The listing builds one solid part. Answer for the finished solid, in the listing's coordinates (mm). A direction names the side the tool comes from. Round coordinates to 2 decimals unless told otherwise and drop trailing zeros. Write each loop counter-clockwise with the first axis right and the second up, starting at its lowest first coordinate (ties: lowest second). Pieces come first, ordered by that corner, then holes.
(1) A cutting plane is placed at C-C, the plane z = -40. Give the vertices of the cut face in (x, y), and give its area (3 significant figures).
(2) A cutting plane is placed at A-A, the plane y = 8. Give the vertices of the cut face in (x, z).
(3) Find the intervals of material crossed by probe 1 along Y at (x, z) = (42.5, 11); probe 2 along Y at (x, z) = (-42.5, -34.5); probe 3 along X at (y, z) = (24.5, 4), in increasing order.
(4) A cutting plane is placed at B-B, the plane z = -11. Give the vertices of the cut face in (x, y).
(5) A cutting plane is placed at D-D, the plane x = 0. Give the vertices of the cut face in (y, z).
(6) Each of these flat-tipped pins is pushed along its axis until it touches: pin 1 Ø6 at (y, z) = (5.5, 10) entering from +X; pin 2 Ø4 at (x, y) = (-41.5, 8) entering from +Z; pin 3 Ø4 at (x, y) = (-38, 13) entering from +Z; pin 4 Ø10.5 at (x, y) = (-44, 24.5) entering from +Z. Where does it stop, or does it pass through?
(7) For faces 4 (the face through (-44, 29.5, -11)), 5 (the face through (9.76, 14.79, 20)), 6 (the face through (36.3, 9.95, 8.31)), determine the directions among +Z, -Z, +X, -X, +Y, -Y from which every point of the face is accessible in a straight line to the end or side of a thin tool.
(8) The mould has two halves that part along Y. Classify faces 1 (the face through (43, 15, 14)), 2 (the face through (36.3, 23.95, 8.31)), 3 (the face through (-42.55, 0.49, 13.73)): +Y half, -Y half, draft (parallel to the pull), parting line (faces both ways), or undercut.
from build123d import *

# Parameters (mm, degrees)
SKETCH1_R               = 32.5
SKETCH1_R_2             = 6
BOSS_EXTRUDE1_DEPTH     = 30
CUT_EXTRUDE1_START      = -0.5
CUT_EXTRUDE1_DEPTH      = 0.5
SKETCH3_R               = 4.5
CUT_EXTRUDE2_DEPTH      = 108.277650829
CUT_EXTRUDE3_DEPTH      = 10
CUT_EXTRUDE3_DEPTH_BACK = 25
SKETCH4_R               = 6.5
FILLET1_R               = 10
CHAMFER1_SIZE           = 1
CHAMFER2_SIZE           = 1


with BuildPart() as part:
    # Sketch1 → Boss-Extrude1 (new body)
    with BuildSketch(Plane(origin=(0, 0, 0), x_dir=(1, 0, 0), z_dir=(0, 1, 0))):
        with BuildLine():
            Line((-34, -23), (-55, -2))
            Line((-55, -2), (-55, 50))
            Line((-55, 50), (55, 50))
            Line((55, 50), (55, -2))
            Line((55, -2), (34, -23))
            ThreePointArc((34, -23), (0, -37.083261121), (-34, -23))
        make_face()
        with Locations(Location((0, 11, 0), (0, 0, 270))):
            Circle(SKETCH1_R, mode=Mode.SUBTRACT)
        with Locations(Location((-30, 40, 0), (0, 0, 90))):
            Circle(SKETCH1_R_2, mode=Mode.SUBTRACT)
    extrude(amount=BOSS_EXTRUDE1_DEPTH)

    # Sketch2 → Cut-Extrude1 (cut)
    with BuildSketch(Plane(origin=(0, 30, 0), x_dir=(1, 0, 0), z_dir=(0, 1, 0)).offset(CUT_EXTRUDE1_START)):
        with BuildLine():
            ThreePointArc((-32.461205211, 9.4125), (-32.490299855, 10.206013022), (-32.5, 11))
            Line((-32.5, 11), (-55, 11))
            Line((-55, 11), (-55, 9.4125))
            Line((-55, 9.4125), (-32.461205211, 9.4125))
        make_face()
        with BuildLine():
            Line((-55, 11), (-32.5, 11))
            ThreePointArc((-32.5, 11), (-32.490299855, 11.793986978), (-32.461205211, 12.5875))
            Line((-32.461205211, 12.5875), (-55, 12.5875))
            Line((-55, 12.5875), (-55, 11))
        make_face()
        with BuildLine():
            Line((55, 11), (32.5, 11))
            ThreePointArc((32.5, 11), (32.490299855, 10.206013022), (32.461205211, 9.4125))
            Line((32.461205211, 9.4125), (55, 9.4125))
            Line((55, 9.4125), (55, 11))
        make_face()
        with BuildLine():
            ThreePointArc((32.461205211, 12.5875), (32.490299855, 11.793986978), (32.5, 11))
            Line((32.5, 11), (55, 11))
            Line((55, 11), (55, 12.5875))
            Line((55, 12.5875), (32.461205211, 12.5875))
        make_face()
    extrude(amount=CUT_EXTRUDE1_DEPTH, mode=Mode.SUBTRACT)

    # Sketch3 → Cut-Extrude2 (cut, through all)
    with BuildSketch(Plane(origin=(0, 0, -50), x_dir=(-1, 0, 0), z_dir=(0, 0, -1))):
        with Locations((42.5, 8)):
            Circle(SKETCH3_R)
        with Locations((-42.5, 8)):
            Circle(SKETCH3_R)
        with Locations((-42.5, 22)):
            Circle(SKETCH3_R)
        with Locations((42.5, 22)):
            Circle(SKETCH3_R)
    extrude(amount=-CUT_EXTRUDE2_DEPTH, mode=Mode.SUBTRACT)

    # Sketch4 → Cut-Extrude3 (cut, two sides: drawn at the far end of the back side and taken through both)
    with BuildSketch(Plane(origin=(0, 0, 10), x_dir=(-1, 0, 0), z_dir=(0, 0, -1)).offset(-CUT_EXTRUDE3_DEPTH_BACK)):
        with Locations((-42.5, 22)):
            Circle(SKETCH4_R)
        with Locations((-42.5, 8)):
            Circle(SKETCH4_R)
        with Locations(Location((42.5, 8, 0), (0, 0, 180))):
            Circle(SKETCH4_R)
        with Locations(Location((42.5, 22, 0), (0, 0, 180))):
            Circle(SKETCH4_R)
    extrude(amount=CUT_EXTRUDE3_DEPTH + CUT_EXTRUDE3_DEPTH_BACK, mode=Mode.SUBTRACT)

    # Fillet1
    fillet1_edges = [part.edges().sort_by_distance(p)[0] for p in [
        (55, 15, 2),
        (-55, 15, 2),
    ]]
    fillet(fillet1_edges, radius=FILLET1_R)

    # Chamfer1
    # the kernel refuses this chamfer: 1 mm, written as the material it takes off along each edge
    with BuildSketch(Plane(origin=(-34, 30, 23), x_dir=(0.7068394360706738, 0.0274958766105857, -0.7068394360706733), z_dir=(-0.7071067811865474, 0, -0.7071067811865478)), Plane(origin=(52.071067812, 30, 4.928932188), x_dir=(-0.7068394360706738, 0.02749587661058558, -0.7068394360706733), z_dir=(-0.7071067811865474, 0, 0.7071067811865478))) as chamfer1_piece_1:
        Polygon((CHAMFER1_SIZE * 0.999621916911, CHAMFER1_SIZE * 0.0274958766106), (-CHAMFER1_SIZE * 0.0274958766106, CHAMFER1_SIZE * 0.999621916911), (0, 0), align=None)
    extrude(amount=25.556349186, mode=Mode.SUBTRACT)
    with BuildSketch(Plane(origin=(55, 30, -11.984182988), x_dir=(-0.9996219169112968, 0.02749587661058555, 0), z_dir=(0, 0, 1)), Plane(origin=(-55, 30, -2.142135624), x_dir=(0.9996219169112968, 0.02749587661058555, 0), z_dir=(0, 0, -1))) as chamfer1_piece_2:
        Polygon((CHAMFER1_SIZE * 0.999621916911, CHAMFER1_SIZE * 0.0274958766106), (-CHAMFER1_SIZE * 0.0274958766106, CHAMFER1_SIZE * 0.999621916911), (0, 0), align=None)
    extrude(amount=9.842047364, mode=Mode.SUBTRACT)
    with BuildSketch(Plane(origin=(45, 30, -2.142135624), x_dir=(1, 0, 0), z_dir=(0, 0, -1))) as chamfer1_piece_3:
        Polygon((10 - CHAMFER1_SIZE, 0), (10, CHAMFER1_SIZE), (10, 0), align=None)
    revolve(axis=Axis((45, 30, -2.142135624), (0, -1, 0)), revolution_arc=45, mode=Mode.SUBTRACT)
    with BuildSketch(Plane(origin=(-45, 30, -2.142135624), x_dir=(-1, 0, 0), z_dir=(0, 0, -1))) as chamfer1_piece_4:
        Polygon((10 - CHAMFER1_SIZE, 0), (10, -CHAMFER1_SIZE), (10, 0), align=None)
    revolve(axis=Axis((-45, 30, -2.142135624), (0, 1, 0)), revolution_arc=45, mode=Mode.SUBTRACT)
    with BuildSketch(Plane(origin=(0, 30, -11), x_dir=(0.7071067811865475, 0, 0.7071067811865475), z_dir=(0.7071067811865475, 0, -0.7071067811865475))) as chamfer1_piece_5:
        Polygon((48.083261121 - CHAMFER1_SIZE, 0), (48.083261121, CHAMFER1_SIZE), (48.083261121, 0), align=None)
    revolve(axis=Axis((0, 30, -11), (0, -1, 0)), revolution_arc=90, mode=Mode.SUBTRACT)
    with BuildSketch(Plane(origin=(55, 30, -52.571682988), x_dir=(0.0274958766105891, -0.9996219169112968, 0), z_dir=(0, 0, 1)), Plane(origin=(-55, 30, -10.015817012), x_dir=(-0.0274958766105891, -0.9996219169112968, 0), z_dir=(0, 0, -1))) as chamfer1_piece_6:
        Polygon((CHAMFER1_SIZE * 0.999621916911, -CHAMFER1_SIZE * 0.0274958766106), (-CHAMFER1_SIZE * 0.0274958766106, -CHAMFER1_SIZE * 0.999621916911), (0, 0), align=None)
    extrude(amount=42.555865976, mode=Mode.SUBTRACT)

    # Chamfer2
    chamfer2_edges = [part.edges().sort_by_distance(p)[0] for p in [
        (-43.035533906, 0, 13.964466094),
        (55, 0, -26.071067812),
        (54.238795325, 0, 1.6846987),
        (-54.238795325, 0, 1.6846987),
        (43.035533906, 0, 13.964466094),
        (0, 0, 37.083261121),
        (-55, 0, -26.071067812),
    ]]
    chamfer(chamfer2_edges, length=CHAMFER2_SIZE)


solid = part.part
Solutions:
1. outline: (-55, 1) - (-54, 0) - (-36, 0) - (-36, 30) - (-54, 30) - (-55, 29) - close; (-24, 0) - (-14.67, 0) - (-14.67, 30) - (-24, 30) - close; (14.67, 0) - (54, 0) - (55, 1) - (55, 29) - (54, 30) - (14.67, 30) - close; hole circle Ø9 at (-42.5, 8); hole circle Ø9 at (-42.5, 22); hole circle Ø9 at (42.5, 8); hole circle Ø9 at (42.5, 22)
1. area: 1,800 mm2
2. outline: (-55, -50) - (-47, -50) - (-47, 0) - (-49, 0) - (-49, 8) - (-52.07, 4.93) arc R10 ccw to (-55, -2.14) - close; (-38, -50) - (38, -50) - (38, 0) - (36, 0) - (36, 21) - (34, 23) arc R48.08 ccw to (-34, 23) - (-36, 21) - (-36, 0) - (-38, 0) - close; (47, -50) - (55, -50) - (55, -2.14) arc R10 ccw to (52.07, 4.93) - (49, 8) - (49, 0) - (47, 0) - close; hole circle Ø12 at (-30, -40); hole circle Ø65 at (0, -11)
3. probe 1: y = 0 to 1.5, 14.5 to 15.5, 28.5 to 30
3. probe 2: y = 0 to 3.5, 12.5 to 17.5, 26.5 to 30
3. probe 3: x = -52.89 to -48.5, -36.5 to -28.83, 28.83 to 36.5, 48.5 to 52.89
4. outline: (-55, 1) - (-54, 0) - (-32.5, 0) - (-32.5, 29.5) - (-54.5, 29.5) - (-55, 29) - close; (32.5, 0) - (54, 0) - (55, 1) - (55, 29) - (54.5, 29.5) - (32.5, 29.5) - close; hole circle Ø9 at (-42.5, 8); hole circle Ø9 at (-42.5, 22); hole circle Ø9 at (42.5, 8); hole circle Ø9 at (42.5, 22)
5. outline: (0, -50) - (30, -50) - (30, -43.5) - (0, -43.5) - close; (0, 21.5) - (30, 21.5) - (30, 36.08) - (29, 37.08) - (1, 37.08) - (0, 36.08) - close
6. pin 1: stops at x = 50
6. pin 2: passes through
6. pin 3: stops at z = 21
6. pin 4: stops at z = 16.86
7. face 4: +X, -X, +Y
7. face 5: +Y, -Y
7. face 6: +Z
8. face 1: draft
8. face 2: undercut
8. face 3: -Y half
